from build123d import *

# Parameters (mm, degrees)
F1_DEPTH    = 14
F2_DEPTH    = 13.5
F0_R        = 9.5
F3_DEPTH    = 9.5
F4_DEPTH    = 9.5
F5_DEPTH    = 28
F0_R_2      = 1.5
F6_DEPTH    = 2.5
F7_SIZE     = 2.2
F8_T1_DEPTH = 50.8601958556
F9_DEPTH    = 9.5
F10_SIZE    = 1.3


# Not quite as in the source:
# - a fillet or chamfer that OpenCascade refuses, or shapes differently, is made with other operations: its cross-section is extruded or revolved along the edge and cut away or added


with BuildPart() as f1:
    # F0 (on Top) → F1 (new body)
    with BuildSketch(Plane.XY):
        Polygon((10, 2.1650635095), (8.75, 2.1650635095), (7.5, 0), (8.75, -2.1650635095), (10, -2.1650635095), (10, 0), align=None)
        Polygon((11.25, 2.1650635095), (10, 2.1650635095), (10, 0), (10, -2.1650635095), (11.25, -2.1650635095), (12.5, 0), align=None)
    extrude(amount=F1_DEPTH)



with BuildPart() as f2:
    # F0 (on Top) → F2 (new body)
    with BuildSketch(Plane.XY):
        with BuildLine():
            ThreePointArc((10, -5), (5, 0), (10, 5))
            Line((10, 5), (10, 6.5))
            ThreePointArc((10, 6.5), (3.5, 0), (10, -6.5))
            Line((10, -6.5), (10, -5))
        make_face()
        with BuildLine():
            Line((10, 6.5), (10, 5))
            ThreePointArc((10, 5), (13.5355339059, 3.5355339059), (15, 0))
            ThreePointArc((15, 0), (13.5355339059, -3.5355339059), (10, -5))
            Line((10, -5), (10, -6.5))
            ThreePointArc((10, -6.5), (14.5961940777, -4.5961940777), (16.5, 0))
            ThreePointArc((16.5, 0), (14.5961940777, 4.5961940777), (10, 6.5))
        make_face()
    extrude(amount=F2_DEPTH)


with BuildPart() as f1_1:
    add(f1.part)

    add(f2.part)  # F3 merges F2
    # F0 (on Top) → F3 (join)
    with BuildSketch(Plane.XY):
        with Locations((10, 0)):
            Circle(F0_R)
        with BuildLine():
            ThreePointArc((10, -6.5), (3.5, 0), (10, 6.5))
            ThreePointArc((10, 6.5), (14.5961940777, 4.5961940777), (16.5, 0))
            ThreePointArc((16.5, 0), (14.5961940777, -4.5961940777), (10, -6.5))
        make_face(mode=Mode.SUBTRACT)
        with BuildLine():
            Line((7.5, 0), (8.75, 2.1650635095))
            Line((8.75, 2.1650635095), (10, 2.1650635095))
            Line((10, 2.1650635095), (10, 5))
            ThreePointArc((10, 5), (5, 0), (10, -5))
            Line((10, -5), (10, -2.1650635095))
            Line((10, -2.1650635095), (8.75, -2.1650635095))
            Line((8.75, -2.1650635095), (7.5, 0))
        make_face()
        with BuildLine():
            Line((10, 5), (10, 2.1650635095))
            Line((10, 2.1650635095), (11.25, 2.1650635095))
            Line((11.25, 2.1650635095), (12.5, 0))
            Line((12.5, 0), (11.25, -2.1650635095))
            Line((11.25, -2.1650635095), (10, -2.1650635095))
            Line((10, -2.1650635095), (10, -5))
            ThreePointArc((10, -5), (13.5355339059, -3.5355339059), (15, 0))
            ThreePointArc((15, 0), (13.5355339059, 3.5355339059), (10, 5))
        make_face()
    extrude(amount=F3_DEPTH)

    # F0 (on Top) → F4 (join)
    with BuildSketch(Plane.XY):
        Polygon((20, 10), (-20, 10), (-20, 8), (-20, 0), (-20, -8), (-20, -10), (20, -10), (20, -8), (20, 0), (20, 8), align=None)
        with BuildLine():
            ThreePointArc((-7.5, 0), (-12.5, -5), (-17.5, 0))
            ThreePointArc((-17.5, 0), (-12.5, 5), (-7.5, 0))
        make_face(mode=Mode.SUBTRACT)
        with Locations((10, 0)):
            Circle(F0_R, mode=Mode.SUBTRACT)
        with Locations((10, 0)):
            Circle(F0_R)
        with BuildLine():
            ThreePointArc((10, -6.5), (3.5, 0), (10, 6.5))
            ThreePointArc((10, 6.5), (14.5961940777, 4.5961940777), (16.5, 0))
            ThreePointArc((16.5, 0), (14.5961940777, -4.5961940777), (10, -6.5))
        make_face(mode=Mode.SUBTRACT)
    extrude(amount=F4_DEPTH)

    # F0 (on Top) → F5 (join)
    with BuildSketch(Plane.XY):
        Polygon((20, 10), (-20, 10), (-20, 8), (-20, 0), (-20, -8), (-20, -10), (20, -10), (20, -8), (20, 0), (20, 8), align=None)
        with BuildLine():
            ThreePointArc((-7.5, 0), (-12.5, -5), (-17.5, 0))
            ThreePointArc((-17.5, 0), (-12.5, 5), (-7.5, 0))
        make_face(mode=Mode.SUBTRACT)
        with Locations((10, 0)):
            Circle(F0_R, mode=Mode.SUBTRACT)
        with Locations((10, 0)):
            Circle(F0_R)
        with BuildLine():
            ThreePointArc((10, -6.5), (3.5, 0), (10, 6.5))
            ThreePointArc((10, 6.5), (14.5961940777, 4.5961940777), (16.5, 0))
            ThreePointArc((16.5, 0), (14.5961940777, -4.5961940777), (10, -6.5))
        make_face(mode=Mode.SUBTRACT)
        Polygon((10, 2.1650635095), (8.75, 2.1650635095), (7.5, 0), (8.75, -2.1650635095), (10, -2.1650635095), (10, 0), align=None)
        Polygon((11.25, 2.1650635095), (10, 2.1650635095), (10, 0), (10, -2.1650635095), (11.25, -2.1650635095), (12.5, 0), align=None)
        with BuildLine():
            Line((7.5, 0), (8.75, 2.1650635095))
            Line((8.75, 2.1650635095), (10, 2.1650635095))
            Line((10, 2.1650635095), (10, 5))
            ThreePointArc((10, 5), (5, 0), (10, -5))
            Line((10, -5), (10, -2.1650635095))
            Line((10, -2.1650635095), (8.75, -2.1650635095))
            Line((8.75, -2.1650635095), (7.5, 0))
        make_face()
        with BuildLine():
            Line((10, 5), (10, 2.1650635095))
            Line((10, 2.1650635095), (11.25, 2.1650635095))
            Line((11.25, 2.1650635095), (12.5, 0))
            Line((12.5, 0), (11.25, -2.1650635095))
            Line((11.25, -2.1650635095), (10, -2.1650635095))
            Line((10, -2.1650635095), (10, -5))
            ThreePointArc((10, -5), (13.5355339059, -3.5355339059), (15, 0))
            ThreePointArc((15, 0), (13.5355339059, 3.5355339059), (10, 5))
        make_face()
        with BuildLine():
            ThreePointArc((10, -5), (5, 0), (10, 5))
            Line((10, 5), (10, 6.5))
            ThreePointArc((10, 6.5), (3.5, 0), (10, -6.5))
            Line((10, -6.5), (10, -5))
        make_face()
        with BuildLine():
            Line((10, 6.5), (10, 5))
            ThreePointArc((10, 5), (13.5355339059, 3.5355339059), (15, 0))
            ThreePointArc((15, 0), (13.5355339059, -3.5355339059), (10, -5))
            Line((10, -5), (10, -6.5))
            ThreePointArc((10, -6.5), (14.5961940777, -4.5961940777), (16.5, 0))
            ThreePointArc((16.5, 0), (14.5961940777, 4.5961940777), (10, 6.5))
        make_face()
        with BuildLine():
            ThreePointArc((-7.5, 0), (-12.5, 5), (-17.5, 0))
            ThreePointArc((-17.5, 0), (-12.5, -5), (-7.5, 0))
        make_face()
    extrude(amount=-F5_DEPTH)

    # F0 (on Top) → F6 (join)
    with BuildSketch(Plane.XY):
        Polygon((28.5, 8), (20, 8), (20, 0), (20, -8), (28.5, -8), align=None)
        with Locations((25.5, -4.5)):
            Circle(F0_R_2, mode=Mode.SUBTRACT)
        with Locations((25.5, 4.5)):
            Circle(F0_R_2, mode=Mode.SUBTRACT)
        Polygon((-20, 0), (-20, 8), (-28.5, 8), (-28.5, -8), (-20, -8), align=None)
        with Locations((-25.5, -4.5)):
            Circle(F0_R_2, mode=Mode.SUBTRACT)
        with Locations((-25.5, 4.5)):
            Circle(F0_R_2, mode=Mode.SUBTRACT)
    extrude(amount=F6_DEPTH)

    # F7
    f7_edges = [f1_1.edges().sort_by_distance(p)[0] for p in [
        (20, 0, 9.5),
    ]]
    chamfer(f7_edges, length=F7_SIZE)

    # F8: chamfer of 6 on 1 edges, made by hand

    # F8_s2 → F8_t1 (cut)
    with BuildSketch(Plane.XZ.offset(-25.4300979278)):
        Polygon((-14, 9.5), (-20, 3.5), (-20, 9.5), align=None)
    extrude(amount=F8_T1_DEPTH, mode=Mode.SUBTRACT)

    # F0 (on Top) → F9 (join)
    with BuildSketch(Plane.XY):
        with BuildLine():
            ThreePointArc((-7.5, 0), (-12.5, 5), (-17.5, 0))
            ThreePointArc((-17.5, 0), (-12.5, -5), (-7.5, 0))
        make_face()
    extrude(amount=F9_DEPTH)

    # F10
    f10_edges = [f1_1.edges().sort_by_distance(p)[0] for p in [
        (20, 0, -28),
        (-20, 0, -28),
    ]]
    chamfer(f10_edges, length=F10_SIZE)


solid = f1_1.part
Work out the finished part from the listing and answer in its coordinate system (mm). A direction names the side the tool comes from. Round coordinates to 2 decimals unless told otherwise and drop trailing zeros. Write each loop counter-clockwise with the first axis right and the second up, starting at its lowest first coordinate (ties: lowest second). Pieces come first, ordered by that corner, then holes.
1) Given pin 1 Ø6 at (y, z) = (-1, -15.5) entering from -X; pin 2 Ø1.5 at (y, z) = (-7, -18.5) entering from +X; pin 3 Ø9.5 at (x, y) = (25.5, -1) entering from +Z; pin 4 Ø2.5 at (x, y) = (25.5, 4.5) entering from +Z, each flat-ended and moving along its own axis, determine where each tip first touches the part or whether it passes through.
2) A cutting plane is placed at D-D (z = -3). Give the vertices of the cut face in (x, y).
3) A cutting plane is placed at B-B (z = 1.5). Give the vertices of the cut face in (x, y).
4) A cutting plane is placed at A-A (x = 25.5). Give the vertices of the cut face in (y, z), plus the area to 3 significant figures.
5) Straight lines are drawn through the part: line 1 (Y direction, x = 25.5, z = 0.75); line 2 (Z direction, x = 6.5, y = -9); line 3 (Z direction, x = -20.5, y = 7.75). For each, find the intervals that lie inside material, in ascending order.
6) A tool of negligible diameter and unlimited length cuts with its end or side. For faces 1 (the flat face through (8.12, -1.07, 11.72)), 2 (the flat face through (24, 0, 0)), 3 (the flat face through (-24, 0, 2.5)), from which of +Z, -Z, +X, -X, +Y, -Y can it reach the whole face along a straight path? Write none if from no direction.
7) The mould has two halves that part along X. Classify faces 4 (the cylindrical face through (-27, -4.43, 1.23)), 5 (the flat face through (24, -8, 1)), 6 (the flat face through (-17.62, 0.14, 5.88)): pulls with the +X half, pulls with the -X half, needs draft (parallel to the pull), parting line crosses it, or undercut.
Completed:
1. pin 1: stops at x = -20
1. pin 2: stops at x = 20
1. pin 3: stops at z = 2.5
1. pin 4: passes through
2. outline: (-20, -10) - (20, -10) - (20, 10) - (-20, 10) - close
3. outline: (-28.5, -8) - (-20, -8) - (-20, -10) - (20, -10) - (20, -8) - (28.5, -8) - (28.5, 8) - (20, 8) - (20, 10) - (-20, 10) - (-20, 8) - (-28.5, 8) - close; hole circle Ø3 at (-25.5, -4.5); hole circle Ø3 at (-25.5, 4.5); hole circle Ø3 at (25.5, -4.5); hole circle Ø3 at (25.5, 4.5)
4. outline: (-8, 0) - (-6, 0) - (-6, 2.5) - (-8, 2.5) - close; (-3, 0) - (3, 0) - (3, 2.5) - (-3, 2.5) - close; (6, 0) - (8, 0) - (8, 2.5) - (6, 2.5) - close
4. area: 25.0 mm2
5. line 1: y = -8 to -6, -3 to 3, 6 to 8
5. line 2: z = -28 to 9.5
5. line 3: z = 0 to 2.5
6. face 1: +Z
6. face 2: -Z, +X, +Y, -Y
6. face 3: +Z, -X, +Y, -Y
7. face 4: undercut
7. face 5: needs draft
7. face 6: pulls with the -X half
